```python
from build123d import *

# Parameters (mm, degrees)
BOSS_EXTRUDE1_DEPTH = 20
CUT_EXTRUDE1_START  = -26
SKETCH2_W           = 16
SKETCH2_H           = 20
SKETCH2_H_2         = 6
CUT_EXTRUDE1_DEPTH  = 26
SKETCH3_R           = 3
CUT_EXTRUDE2_DEPTH  = 2.000000064


with BuildPart() as part:
    # Sketch1 → Boss-Extrude1 (new body)
    with BuildSketch(Plane.XY):
        Polygon((0, 0), (0, 28), (8, 28), (8, 20), (20, 8), (28, 8), (28, 0), align=None)
    extrude(amount=BOSS_EXTRUDE1_DEPTH)

    # Sketch2 → Cut-Extrude1 (cut)
    with BuildSketch(Plane(origin=(28, 0, 0), x_dir=(0, 0, -1), z_dir=(1, 0, 0)).offset(CUT_EXTRUDE1_START)):
        with Locations((-10, 18)):
            Rectangle(SKETCH2_W, SKETCH2_H)
        with Locations((-10, 5)):
            Rectangle(SKETCH2_W, SKETCH2_H_2)
    extrude(amount=CUT_EXTRUDE1_DEPTH, mode=Mode.SUBTRACT)

    # Sketch3 → Cut-Extrude2 (cut)
    with BuildSketch(Plane(origin=(2.000000064, 0, 0), x_dir=(0, 0, -1), z_dir=(1, 0, 0))):
        with Locations((-10, 18)):
            Circle(SKETCH3_R)
        with BuildLine():
            ThreePointArc((-10, 15), (-12.121320344, 15.878679656), (-13, 18))
            Line((-13, 18), (-13, 12))
            ThreePointArc((-13, 12), (-12.121320344, 14.121320344), (-10, 15))
        make_face()
        with BuildLine():
            Line((-7, 12), (-7, 18))
            ThreePointArc((-7, 18), (-7.878679656, 15.878679656), (-10, 15))
            ThreePointArc((-10, 15), (-7.878679656, 14.121320344), (-7, 12))
        make_face()
        with Locations((-10, 12)):
            Circle(SKETCH3_R)
    cut_extrude2 = extrude(amount=-CUT_EXTRUDE2_DEPTH, mode=Mode.SUBTRACT)

    # Mirror2: Cut-Extrude2 across plane
    add(cut_extrude2.mirror(Plane(origin=(0, 0, 0), x_dir=(0, 0, 1), z_dir=(0.7071067811865438, -0.7071067811865512, 0))), mode=Mode.SUBTRACT)


solid = part.part
```
Work out the finished part from the listing and answer in its coordinate system (mm). A direction names the side the tool comes from. Give positions to 0.01 mm unless a question says otherwise; leave off trailing zeros. Write each loop counter-clockwise with the first axis right and the second up, starting at its lowest first coordinate (ties: lowest second). Pieces come first, ordered by that corner, then holes. Notation, with made-up numbers: (35.5, -10) -> (47.5, -10) arc R34 cw to (47.5, 27) -> close; hole circle Ø2 at (2, -16.75). An arc over 180 degrees is marked (long way). Write item = value, one per line.
Q1. Section A-A on z = 10 is taken. Determine the outline of the cut face in (x, y).
Computed values:
outline = (0, 0) -> (9, 0) -> (9, 2) -> (2, 2) -> (2, 9) -> (0, 9) -> close; (0, 21) -> (2, 21) -> (2, 28) -> (0, 28) -> close; (21, 0) -> (28, 0) -> (28, 2) -> (21, 2) -> close
Q2. Flat-ended cylindrical pins translate along their axes: pin 1 Ø5 at (x, z) = (14, 6.5) entering from +Y; pin 2 Ø1 at (x, y) = (14.5, 1) entering from -Z; pin 3 Ø1 at (y, z) = (23.5, 19) entering from +X; pin 4 Ø2 at (x, z) = (23, 19) entering from +Y. Find the tip coordinate at first contact, or state that the pin passes through.
Computed values:
pin_1 = 2
pin_2 = 0
pin_3 = 8
pin_4 = 8
Q3. Section B-B on y = 14.5 is taken. Determine the outline of the cut face in (x, z).
Computed values:
outline = (0, 0) -> (13.5, 0) -> (13.5, 2) -> (2, 2) -> (2, 7) -> (0, 7) -> close; (0, 13) -> (2, 13) -> (2, 18) -> (13.5, 18) -> (13.5, 20) -> (0, 20) -> close
Q4. Consider line 1 along Z through (x, y) = (2.5, 25.5); line 2 along Y through (x, z) = (24.5, 19.25); line 3 along X through (y, z) = (20.75, 12.75). Determine where each line is inside the solid, lowest interval first.
Computed values:
line_1 = 0 to 2, 18 to 20
line_2 = 0 to 8
line_3 = 0 to 2
Q5. Section C-C on x = 26 is taken. Determine the outline of the cut face in (y, z), and give its area (3 significant figures).
Computed values:
outline = (0, 0) -> (8, 0) -> (8, 2) -> (2, 2) -> (2, 18) -> (8, 18) -> (8, 20) -> (0, 20) -> close
area = 64.0 mm^2
Q6. A tool of negligible diameter and unlimited length cuts with its end or side. For faces 1 (the flat face through (1, 15, 7)), 2 (the flat face through (15, 1, 7)), 3 (the flat face through (2, 15, 14)), from which of +Z, -Z, +X, -X, +Y, -Y can it reach the whole face along a straight path? Write none if from no direction.
Computed values:
face_1 = +X, -X
face_2 = +Y, -Y
face_3 = +X, +Y
Q7. For a pull along X with two mould halves and no side action, classify faces 4 (the flat face through (11, 11, 0)), 5 (the flat face through (14, 14, 1)), 6 (the cylindrical face through (9, 1, 10)), 7 (the flat face through (0, 14, 5)) as pulls with the +X half, pulls with the -X half, needs draft (parallel to the pull), parting line crosses it, or undercut.
Computed values:
face_4 = needs draft
face_5 = pulls with the +X half
face_6 = undercut
face_7 = pulls with the -X half
